from build123d import *

# Parameters (mm, degrees)
F0_W        = 36
F0_H        = 36
F0_R        = 1.625
F1_DEPTH    = 1.5
F2_R        = 2
F3_T1_DEPTH = 3.5843159378
F3_T3_DEPTH = 3.5765382717


# Not quite as in the source:
# - a fillet or chamfer that OpenCascade refuses, or shapes differently, is made with other operations: its cross-section is extruded or revolved along the edge and cut away or added


with BuildPart() as f1:
    # F0 (on Top) → F1 (new body)
    with BuildSketch(Plane.XY):
        with Locations((18, -18)):
            Rectangle(F0_W, F0_H)
        with Locations((2.75, -33.25)):
            Circle(F0_R, mode=Mode.SUBTRACT)
        with Locations((33.25, -33.25)):
            Circle(F0_R, mode=Mode.SUBTRACT)
        with BuildLine():
            ThreePointArc((21.7779175478, -11.3763919814), (22.046238649, -11.6387988402), (22.2963811606, -11.918588577))
            ThreePointArc((22.2963811606, -11.918588577), (23.2607600241, -13.5926773143), (23.5988556823, -15.4948579101))
            ThreePointArc((23.5988556823, -15.4948579101), (22.0425607669, -20.1541714045), (18.3719356765, -23.4187950503))
            ThreePointArc((18.3719356765, -23.4187950503), (18.1854087753, -23.510113363), (17.9969356765, -23.5973441498))
            ThreePointArc((17.9969356765, -23.5973441498), (17.8078713111, -23.5092095417), (17.6207740645, -23.4169725439))
            ThreePointArc((17.6207740645, -23.4169725439), (13.9590716003, -20.150973111), (12.3987158352, -15.4990802577))
            ThreePointArc((12.3987158352, -15.4990802577), (12.7360960776, -13.5946679159), (13.7011902766, -11.9185996051))
            ThreePointArc((13.7011902766, -11.9185996051), (13.9513320879, -11.638809208), (14.2196525358, -11.3764016446))
            ThreePointArc((14.2196525358, -11.3764016446), (17.9987831657, -9.9089991809), (21.7779175478, -11.3763919814))
        make_face(mode=Mode.SUBTRACT)
        with Locations((2.75, -2.75)):
            Circle(F0_R, mode=Mode.SUBTRACT)
        with Locations((33.25, -2.75)):
            Circle(F0_R, mode=Mode.SUBTRACT)
        with BuildLine():
            ThreePointArc((18.3719356765, -22.8064015707), (21.6418869825, -19.7559203536), (22.9988556823, -15.4948579101))
            ThreePointArc((22.9988556823, -15.4948579101), (22.7058670076, -13.8225937813), (21.8702080342, -12.3447630196))
            ThreePointArc((21.8702080342, -12.3447630196), (21.6219028277, -12.0632376766), (21.3531767506, -11.8011340904))
            ThreePointArc((21.3531767506, -11.8011340904), (17.9987795183, -10.508999181), (14.644381672, -11.8011324963))
            ThreePointArc((14.644381672, -11.8011324963), (14.3756554704, -12.0632359548), (14.12735013, -12.3447611798))
            ThreePointArc((14.12735013, -12.3447611798), (13.2916900536, -13.8225926629), (12.9987009782, -15.4948579101))
            ThreePointArc((12.9987009782, -15.4948579101), (14.3541308063, -19.7551514484), (17.6219356765, -22.8061746181))
            ThreePointArc((17.6219356765, -22.8061746181), (17.8082968783, -22.9039932616), (17.9969356765, -22.9973441498))
            ThreePointArc((17.9969356765, -22.9973441498), (18.1855728443, -22.9041061909), (18.3719356765, -22.8064015707))
        make_face()
        with BuildLine():
            ThreePointArc((13.7508900496, -15.5000002377), (16.4147091349, -16.5221024247), (17.2508900496, -19.2500002377))
            ThreePointArc((17.2508900496, -19.2500002377), (14.7355024037, -18.3769724477), (13.7124911572, -15.9187616104))
            ThreePointArc((13.7124911572, -15.9187616104), (13.7249235892, -15.7087604135), (13.7508900496, -15.5000002377))
        make_face(mode=Mode.SUBTRACT)
        with BuildLine():
            ThreePointArc((18.7512718965, -19.25059231), (19.5857343833, -16.5222080691), (22.2488645533, -15.4984180975))
            ThreePointArc((22.2488645533, -15.4984180975), (21.4144020665, -18.2268023385), (18.7512718965, -19.25059231))
        make_face(mode=Mode.SUBTRACT)
        with BuildLine():
            Line((18.3719356765, -23.2973441498), (18.3719356765, -22.8064015707))
            ThreePointArc((18.3719356765, -22.8064015707), (18.1855728443, -22.9041061909), (17.9969356765, -22.9973441498))
            ThreePointArc((17.9969356765, -22.9973441498), (17.8082968783, -22.9039932616), (17.6219356765, -22.8061746181))
            Line((17.6219356765, -22.8061746181), (17.6219356765, -23.2973441498))
            Line((17.6219356765, -23.2973441498), (17.6207740645, -23.4169725439))
            ThreePointArc((17.6207740645, -23.4169725439), (17.8078713111, -23.5092095417), (17.9969356765, -23.5973441498))
            ThreePointArc((17.9969356765, -23.5973441498), (18.1854087753, -23.510113363), (18.3719356765, -23.4187950503))
            Line((18.3719356765, -23.4187950503), (18.3719356765, -23.2973441498))
        make_face()
        with BuildLine():
            ThreePointArc((21.3531767506, -11.8011340904), (21.6219028277, -12.0632376766), (21.8702080342, -12.3447630196))
            Line((21.8702080342, -12.3447630196), (22.1000614519, -12.114908892))
            Line((22.1000614519, -12.114908892), (22.2963811606, -11.918588577))
            ThreePointArc((22.2963811606, -11.918588577), (22.046238649, -11.6387988402), (21.7779175478, -11.3763919814))
            Line((21.7779175478, -11.3763919814), (21.5697305471, -11.5845796251))
            Line((21.5697305471, -11.5845796251), (21.3531767506, -11.8011340904))
        make_face()
        with BuildLine():
            ThreePointArc((14.12735013, -12.3447611798), (14.3756554704, -12.0632359548), (14.644381672, -11.8011324963))
            Line((14.644381672, -11.8011324963), (14.4278279784, -11.584577928))
            Line((14.4278279784, -11.584577928), (14.2196525358, -11.3764016446))
            ThreePointArc((14.2196525358, -11.3764016446), (13.9513320879, -11.638809208), (13.7011902766, -11.9185996051))
            Line((13.7011902766, -11.9185996051), (13.8974968216, -12.114906943))
            Line((13.8974968216, -12.114906943), (14.12735013, -12.3447611798))
        make_face()
    extrude(amount=F1_DEPTH)

    # F2
    f2_edges = [f1.edges().sort_by_distance(p)[0] for p in [
        (36, -36, 0.75),
        (0, -36, 0.75),
        (36, 0, 0.75),
        (0, 0, 0.75),
    ]]
    fillet(f2_edges, radius=F2_R)

    # F3: fillet of radius 4 on 2 edges, made by hand

    # F3_s2 → F3_t1 (cut)
    with BuildSketch(Plane.XY.offset(-1.0421579689)):
        with BuildLine():
            ThreePointArc((22.982065791, -15.7463315161), (22.9951448823, -15.4123328014), (22.980292521, -15.0784082419))
            ThreePointArc((22.980292521, -15.0784082419), (22.9939159673, -15.2864395382), (22.9988556823, -15.4948579101))
            ThreePointArc((22.9988556823, -15.4948579101), (22.9913576348, -15.6206545954), (22.982065791, -15.7463315161))
        make_face()
    extrude(amount=F3_T1_DEPTH, mode=Mode.SUBTRACT)

    # F3_s4 → F3_t3 (cut)
    with BuildSketch(Plane.XY.offset(-1.0382691359)):
        with BuildLine():
            ThreePointArc((13.0171302774, -15.0799593578), (13.0023850075, -15.4126416016), (13.0153633645, -15.745397459))
            ThreePointArc((13.0153633645, -15.745397459), (13.0061419392, -15.6201868903), (12.9987009782, -15.4948579101))
            ThreePointArc((12.9987009782, -15.4948579101), (13.0036060893, -15.2872172094), (13.0171302774, -15.0799593578))
        make_face()
    extrude(amount=F3_T3_DEPTH, mode=Mode.SUBTRACT)


solid = f1.part
The model under review builds one solid part; all positions refer to its coordinate system, in mm. A direction names the side the tool comes from. Give positions to 0.01 mm unless a question says otherwise; leave off trailing zeros. Order: outer loops, then holes, each group sorted by start corner. A loop starts at its lowest first (then second) coordinate and runs counter-clockwise, first axis right, second up. Notation, with made-up numbers: (-5, -35) -> (15, -35) arc R13 cw to (15, -27) -> close; hole circle Ø5 at (-5.75, 57). An arc over 180 degrees is marked (long way). Write item = value, one per line. Start each with the question number.
(1) Take a section at A-A (y = -33.25). Write out the cut boundary in (x, z) (3 decimals), plus the area to 4 significant figures.
(2) Take a section at C-C (z = 1). State how many separate pieces and enclosed holes the cut face has, plus the area to 3 significant figures.
(3) Tool access review of faces 1 (the cylindrical face through (0.57, -0.6, 0.76)), 2 (the cylindrical face through (18.05, -10.51, 0.74)): name each direction out of +Z, -Z, +X, -X, +Y, -Y from which nothing blocks a thin tool from reaching the whole face with its end or side.
(4) For pin 1 Ø3 at (x, y) = (2.75, -2.75) entering from +Z; pin 2 Ø4 at (x, y) = (33.25, -33.25) entering from +Z, all flat-tipped, find the tip position at first contact; note any pin that passes through.
(5) Draft analysis for pull direction Y (two halves, no side actions). For faces 3 (the cylindrical face through (0.57, -35.4, 0.76)), 4 (the cylindrical face through (14, -20.21, 0.74)), 5 (the flat face through (18, -18, 1.5)), state which applies: +Y half, -Y half, draft (parallel to the pull), parting line (faces both ways), or undercut.
(6) Take a section at B-B (x = 33.25). Write out the cut boundary in (y, z) (3 decimals), plus the area to 4 significant figures.
(7) For L1, parallel to Y at x = 33.25, z = 0.55 (3 decimals); L2, parallel to Y at x = 2, z = 0.95; L3, parallel to X at y = -14.5, z = 1.45, list the stretches that pass through material, from the lowest coordinate up. Write a range as from..to.
Returned:
q1.outline = (0, 0) -> (1.125, 0) -> (1.125, 1.5) -> (0, 1.5) -> close; (4.375, 0) -> (31.625, 0) -> (31.625, 1.5) -> (4.375, 1.5) -> close; (34.875, 0) -> (36, 0) -> (36, 1.5) -> (34.875, 1.5) -> close
q1.area = 44.25 mm²
q2.separate_pieces = 1
q2.enclosed_holes = 9
q2.area = 1,220 mm²
q3.face_1 = +Z, -Z, -X, +Y
q3.face_2 = +Z, -Z
q4.pin_1 = through
q4.pin_2 = 1.5
q5.face_3 = -Y half
q5.face_4 = undercut
q5.face_5 = draft
q6.outline = (-36, 0) -> (-34.875, 0) -> (-34.875, 1.5) -> (-36, 1.5) -> close; (-31.625, 0) -> (-4.375, 0) -> (-4.375, 1.5) -> (-31.625, 1.5) -> close; (-1.125, 0) -> (0, 0) -> (0, 1.5) -> (-1.125, 1.5) -> close
q6.area = 44.25 mm²
q7.L1 = -36..-34.875, -31.625..-4.375, -1.125..0
q7.L2 = -36..-34.69, -31.81..-4.19, -1.31..0
q7.L3 = 0..12.49, 13.1..22.9, 23.51..36
